from build123d import *


with BuildPart() as part:
    # Sketch1 → Revolve1 (revolve)
    with BuildSketch(Plane(origin=(0, 0, 0), x_dir=(0, 0, -1), z_dir=(1, 0, 0)), mode=Mode.PRIVATE) as revolve1_sk:
        with BuildLine():
            Line((-27.75, 0), (-27.75, -1.5))
            Line((-27.75, -1.5), (-26.75, -1.5))
            Line((-26.75, -1.5), (-26.75, -11.5))
            Line((-26.75, -11.5), (-25.75, -11.5))
            Line((-25.75, -11.5), (-22.796999799, -28.247296355))
            ThreePointArc((-22.796999799, -28.247296355), (-22.112959512, -29.432088886), (-20.827384293, -29.9))
            Line((-20.827384293, -29.9), (0, -29.9))
            Line((0, -29.9), (0, -32.4))
            Line((0, -32.4), (-19.936900461, -32.4))
            ThreePointArc((-19.936900461, -32.4), (-32.760664046, -19.338533844), (-38, -1.8))
            Line((-38, -1.8), (-35, -1.8))
            Line((-35, -1.8), (-35, 8.2))
            Line((-35, 8.2), (-27.75, 8.2))
            Line((-27.75, 8.2), (-27.75, 0))
        make_face()
    revolve(revolve1_sk.sketch.rotate(Axis((0, 0, 0), (0, 1, 0)), 180), axis=Axis((0, 0, 0), (0, 1, 0)))


solid = part.part
Source: CAD feature listing. Evaluate the final solid. Frame: model axes, mm. A direction names the side the tool comes from. Round coordinates to 2 decimals unless told otherwise and drop trailing zeros. Write each loop counter-clockwise with the first axis right and the second up, starting at its lowest first coordinate (ties: lowest second). Pieces come first, ordered by that corner, then holes. Notation, with made-up numbers: M 56,-28 L 98,-28 A30 cw 98,11 Z; hole C 15.5,80 d6. An arc over 180 degrees is marked long. One line per item, written item: value. Start each with the question number.
Item 1: Section query C-C (z = 29.5). Return the cut outline in (x, y), plus the area to 3 significant figures.
Item 2: Section query B-B (y = -19). Return the cut outline in (x, z), plus the area to 3 significant figures.
Item 3: Section query D-D (y = -13.5). Return the cut outline in (x, z).
Item 4: Pin query (flat end, axial travel): pin 1 (2 mm diameter, centred on x = -21.5, z = -12.5, fed in from +Y); pin 2 (5 mm diameter, centred on x = 16, z = -8.5, fed in from +Y); pin 3 (2 mm diameter, centred on y = -21, z = 29.5, fed in from -X). Return the tip coordinate at first contact, or that it passes through.
Item 5: Set-up query: faces 5 (the flat face through (0, -32.4, 0)), 6 (the cylindrical face through (-8.335, 3.282, -26.469)). Return all of +Z, -Z, +X, -X, +Y, -Y with unobstructed straight access to the full face (end or side cutting, diameter ignored); none if empty.
Item 6: Ray query, L1, parallel to Z at x = 3.5, y = 0; L2, parallel to X at y = 0, z = -11; L3, parallel to Y at x = -11, z = -1. Return the intervals inside material, ascending. Write a range as from..to.
Item 7: Mould query, pull axis Z, two halves, no side actions, for faces 1 (the cylindrical face through (34.168, 3.27, 7.587)), 2 (the flat face through (-15, -1.5, 23)), 3 (the cylindrical face through (16.277, -6.57, 21.228)), 4 (the flat face through (-26, 8.2, 11)). Classes: pulls with the +Z half, pulls with the -Z half, needs draft (parallel to the pull), parting line crosses it, or undercut.
Item 8: Section query A-A (x = 0). Return the cut outline in (y, z).
Result set:
1. outline: M -23.95,-1.8 A24.02 ccw 23.95,-1.8 L 18.83,-1.8 L 18.83,8.2 L -18.83,8.2 L -18.83,-1.8 Z
1. area: 1,200 mm²
2. outline: C 0,0 d65.92; hole C 0,0 d48.86
2. area: 1,540 mm²
3. outline: C 0,0 d71.13; hole C 0,0 d50.79
4. pin 1: stops at y = -11.5
4. pin 2: stops at y = -29.9
4. pin 3: stops at x = -14.4
5. face 5: +Z, -Z, +X, -X, -Y
5. face 6: +Y
6. L1: z = -34.82..-27.53, 27.53..34.82
6. L2: x = -33.23..-25.48, 25.48..33.23
6. L3: y = -32.4..-29.9
7. face 1: parting line crosses it
7. face 2: undercut
7. face 3: undercut
7. face 4: needs draft
8. outline: M -32.4,-19.94 A38.04 ccw -1.8,-38 L -1.8,-35 L 8.2,-35 L 8.2,-27.75 L -1.5,-27.75 L -1.5,-26.75 L -11.5,-26.75 L -11.5,-25.75 L -28.25,-22.8 A2 cw -29.9,-20.83 L -29.9,20.83 A2 cw -28.25,22.8 L -11.5,25.75 L -11.5,26.75 L -1.5,26.75 L -1.5,27.75 L 8.2,27.75 L 8.2,35 L -1.8,35 L -1.8,38 A38.04 ccw -32.4,19.94 Z
